```python
from build123d import *

# Parameters (mm, degrees)
IZIM1_R                     = 18
Y_KSEKLIK_EKSTR_ZYON1_DEPTH = 380
RADYUS1_R                   = 100
RADYUS2_R                   = 30


with BuildPart() as part:
    # Çizim1 → Yükseklik-Ekstrüzyon1 (new body)
    with BuildSketch(Plane.XY):
        with BuildLine():
            Line((-28, 0), (-28, 30))
            Line((-28, 30), (-178, 30))
            Line((-178, 30), (-178, 48))
            Line((-178, 48), (622, 48))
            Line((622, 48), (622, 30))
            Line((622, 30), (472, 30))
            Line((472, 30), (472, 0))
            ThreePointArc((472, 0), (444, -28), (416, 0))
            Line((416, 0), (416, 30))
            Line((416, 30), (28, 30))
            Line((28, 30), (28, 0))
            ThreePointArc((28, 0), (0, -28), (-28, 0))
        make_face()
        Circle(IZIM1_R, mode=Mode.SUBTRACT)
        with Locations((444, 0)):
            Circle(IZIM1_R, mode=Mode.SUBTRACT)
    extrude(amount=Y_KSEKLIK_EKSTR_ZYON1_DEPTH)

    # Radyus1
    radyus1_edges = [part.edges().sort_by_distance(p)[0] for p in [
        (-178, 39, 0),
        (-178, 39, 380),
    ]]
    fillet(radyus1_edges, radius=RADYUS1_R)

    # Radyus2
    radyus2_edges = [part.edges().sort_by_distance(p)[0] for p in [
        (622, 39, 0),
        (622, 39, 380),
    ]]
    fillet(radyus2_edges, radius=RADYUS2_R)


solid = part.part
```
CAD build for the part. Positions are in the model's coordinates, mm. A direction names the side the tool comes from. Coordinates: 2 decimals unless noted, no trailing zeros. Write each loop counter-clockwise with the first axis right and the second up, starting at its lowest first coordinate (ties: lowest second). Pieces come first, ordered by that corner, then holes. Notation, with made-up numbers: (42, 13) -> (59, 13) arc R17 ccw to (59, 40) -> close; hole circle Ø9 at (87.25, -25). An arc over 180 degrees is marked (long way). Return JSON: item names as keys, results as strings. Group by question number.
Q1. Flat gauge pins, fed straight in: pin 1 (4 mm diameter, centred on y = 22.5, z = 238.5, fed in from +X); pin 2 (1.5 mm diameter, centred on y = 9.5, z = 174.5, fed in from -X); pin 3 (4 mm diameter, centred on x = -91.5, z = 51, fed in from -Y). Where does each tip first touch, or does it go through?
Q2. Which spindle directions (+Z, -Z, +X, -X, +Y, -Y) get a long thin tool onto all of the face, cutting with end or side? Do faces 4 (the face through (28, 15, 187)), 5 (the face through (-102, 30, 187)), 6 (the face through (472, 15, 187)). Say none if no direction does.
Q3. Cut at C-C, the plane z = 331. Give the cut face in (x, y), then the cut area to 3 significant figures.
Q4. Pull direction Y, two halves, no side cores. Call faces 1 (the face through (-2.343, 17.847, 187.34)), 2 (the face through (416, 15, 187)), 3 (the face through (0.616, -27.993, 187.34)): released by +Y, released by -Y, zero draft, split by the parting line, or undercut.
Q5. Cut at B-B, the plane z = 188.5. Give the cut face in (x, y).
Q6. Drill centre lines: line 1 (X direction, y = -7, z = 324); line 2 (X direction, y = 18.5, z = 88); line 3 (Y direction, x = 0, z = 167). Where is each one in solid material? Low to high.
Q7. Cut at A-A, the plane x = 0. Give the cut face in (y, z), then the cut area to 3 significant figures.
Returned:
{
 "1": {"pin 1": "stops at x = 472", "pin 2": "stops at x = -28", "pin 3": "stops at y = 30"},
 "2": {"face 4": "+Z, -Z, -Y", "face 5": "+Z, -Z, -X, -Y", "face 6": "+Z, -Z, +X, -Y"},
 "3": {"outline": "(-164.02, 30) -> (-28, 30) -> (-28, 0) arc R28 ccw to (28, 0) -> (28, 30) -> (416, 30) -> (416, 0) arc R28 ccw to (472, 0) -> (472, 30) -> (622, 30) -> (622, 48) -> (-164.02, 48) -> close; hole circle Ø36 at (0, 0); hole circle Ø36 at (444, 0)", "area": "17,900 mm2"},
 "4": {"face 1": "undercut", "face 2": "zero draft", "face 3": "released by -Y"},
 "5": {"outline": "(-178, 30) -> (-28, 30) -> (-28, 0) arc R28 ccw to (28, 0) -> (28, 30) -> (416, 30) -> (416, 0) arc R28 ccw to (472, 0) -> (472, 30) -> (622, 30) -> (622, 48) -> (-178, 48) -> close; hole circle Ø36 at (0, 0); hole circle Ø36 at (444, 0)"},
 "6": {"line 1": "x = -27.11 to -16.58, 16.58 to 27.11, 416.89 to 427.42, 460.58 to 471.11", "line 2": "x = -28 to 28, 416 to 472", "line 3": "y = -28 to -18, 18 to 48"},
 "7": {"outline": "(-28, 0) -> (-18, 0) -> (-18, 380) -> (-28, 380) -> close; (18, 0) -> (48, 0) -> (48, 380) -> (18, 380) -> close", "area": "15,200 mm2"}
}
